```python
from build123d import *

# Parameters (mm, degrees)
SKETCH1_W           = 50
SKETCH1_H           = 53
BOSS_EXTRUDE1_DEPTH = 0.75
BOSS_EXTRUDE2_DEPTH = 1.5
SKETCH7_R           = 2
SKETCH7_R_2         = 1.948313055
CUT_EXTRUDE1_DEPTH  = 39.581083448
SKETCH8_W           = 21
SKETCH8_H           = 2.5
SKETCH8_W_2         = 6
SKETCH8_H_2         = 21
SKETCH8_W_3         = 16
BOSS_EXTRUDE3_DEPTH = 9
SKETCH9_R           = 2
BOSS_EXTRUDE4_DEPTH = 6
SKETCH10_W          = 14.5
SKETCH10_H          = 9
BOSS_EXTRUDE5_DEPTH = 11
SKETCH11_W          = 10
SKETCH11_H          = 7
BOSS_EXTRUDE6_DEPTH = 4
SKETCH12_W          = 6
SKETCH12_H          = 8
BOSS_EXTRUDE7_DEPTH = 6
SKETCH13_W          = 5
SKETCH13_H          = 12
BOSS_EXTRUDE8_DEPTH = 8
FILLET4_R           = 1
FILLET5_R           = 1


with BuildPart() as part:
    # Sketch1 → Boss-Extrude1 (new, symmetric)
    with BuildSketch(Plane(origin=(0, 0, 0), x_dir=(1, 0, 0), z_dir=(0, 1, 0))):
        Rectangle(SKETCH1_W, SKETCH1_H)
    extrude(amount=BOSS_EXTRUDE1_DEPTH, both=True)


with BuildPart() as body_2:
    # Sketch3 → Boss-Extrude2 (new body)
    with BuildSketch(Plane(origin=(0, 0.75, 0), x_dir=(1, 0, 0), z_dir=(0, 1, 0))):
        Polygon((25, -22.246887694), (25, 14.753112306), (28, 13.047029226), (28, -19.952970774), align=None)
    extrude(amount=-BOSS_EXTRUDE2_DEPTH)


with BuildPart() as cut_extrude1_tool:
    # Sketch7 → Cut-Extrude1 (new, through all)
    with BuildSketch(Plane(origin=(0, 0.75, 0), x_dir=(1, 0, 0), z_dir=(0, 1, 0))):
        with Locations(Location((-22.5, 24, 0), (0, 0, 270))):
            Circle(SKETCH7_R)
        with Locations(Location((-22.5, -24, 0), (0, 0, 270))):
            Circle(SKETCH7_R)
        with Locations((25, 11.753112306)):
            Circle(SKETCH7_R_2)
        with Locations((25, -19.246887694)):
            Circle(SKETCH7_R)
    extrude(amount=-CUT_EXTRUDE1_DEPTH)


with BuildPart() as part_1:
    add(part.part)

    # Cut-Extrude1: cut by cut_extrude1_tool
    add(cut_extrude1_tool.part, mode=Mode.SUBTRACT)



with BuildPart() as body_2_1:
    add(body_2.part)

    # Cut-Extrude1: cut by cut_extrude1_tool
    add(cut_extrude1_tool.part, mode=Mode.SUBTRACT)


with BuildPart() as part_2:
    add(part_1.part)

    add(body_2_1.part)  # Boss-Extrude3 merges body 2
    # Sketch8 → Boss-Extrude3 (add)
    with BuildSketch(Plane(origin=(0, 0.75, 0), x_dir=(1, 0, 0), z_dir=(0, 1, 0))):
        with Locations((13.5, 24.25)):
            Rectangle(SKETCH8_W, SKETCH8_H)
        with Locations((-8.5, 24.25)):
            Rectangle(SKETCH8_W, SKETCH8_H)
        with Locations((24, -5)):
            Rectangle(SKETCH8_W_2, SKETCH8_H_2)
        with Locations((15, -24.25)):
            Rectangle(SKETCH8_W_3, SKETCH8_H)
        with Locations((-3, -24.25)):
            Rectangle(SKETCH8_W_3, SKETCH8_H)
    extrude(amount=BOSS_EXTRUDE3_DEPTH)

    # Sketch9 → Boss-Extrude4 (add)
    with BuildSketch(Plane(origin=(0, 0.75, 0), x_dir=(1, 0, 0), z_dir=(0, 1, 0))):
        with Locations(Location((-2, -19, 0), (0, 0, 270))):
            Circle(SKETCH9_R)
        with Locations(Location((-2, -14.5, 0), (0, 0, 270))):
            Circle(SKETCH9_R)
        with Locations(Location((-8, -14.5, 0), (0, 0, 270))):
            Circle(SKETCH9_R)
    extrude(amount=BOSS_EXTRUDE4_DEPTH)

    # Sketch10 → Boss-Extrude5 (add)
    with BuildSketch(Plane(origin=(0, 0.75, 0), x_dir=(1, 0, 0), z_dir=(0, 1, 0))):
        with Locations((-20.75, -14)):
            Rectangle(SKETCH10_W, SKETCH10_H)
    extrude(amount=BOSS_EXTRUDE5_DEPTH)

    # Sketch11 → Boss-Extrude6 (add)
    with BuildSketch(Plane(origin=(0, 0.75, 0), x_dir=(1, 0, 0), z_dir=(0, 1, 0))):
        with Locations((-21, -1)):
            Rectangle(SKETCH11_W, SKETCH11_H)
    extrude(amount=BOSS_EXTRUDE6_DEPTH)

    # Sketch12 → Boss-Extrude7 (add)
    with BuildSketch(Plane(origin=(0, 0.75, 0), x_dir=(1, 0, 0), z_dir=(0, 1, 0))):
        with Locations((-21, 11.5)):
            Rectangle(SKETCH12_W, SKETCH12_H)
    extrude(amount=BOSS_EXTRUDE7_DEPTH)

    # Sketch13 → Boss-Extrude8 (add)
    with BuildSketch(Plane(origin=(0, 0.75, 0), x_dir=(1, 0, 0), z_dir=(0, 1, 0))):
        with Locations((-8.5, 8.5)):
            Rectangle(SKETCH13_W, SKETCH13_H)
    extrude(amount=BOSS_EXTRUDE8_DEPTH)

    # Fillet4
    fillet4_edges = [part_2.edges().sort_by_distance(p)[0] for p in [
        (-25, 0, -26.5),
    ]]
    fillet(fillet4_edges, radius=FILLET4_R)

    # Fillet5
    fillet5_edges = [part_2.edges().sort_by_distance(p)[0] for p in [
        (-25, 0, 26.5),
    ]]
    fillet(fillet5_edges, radius=FILLET5_R)


solid = part_2.part
```
Can you work these out from the model? Positions are in its coordinate system, mm. A direction names the side the tool comes from. Round coordinates to 2 decimals unless told otherwise and drop trailing zeros. Loops run counter-clockwise (first coordinate to the right, second up) from the corner with the lowest first, then second, coordinate; pieces in that order, holes last. Notation, with made-up numbers: (0, 63.5) -> (29, 63.5) arc R30 ccw to (29, 102.5) -> close; hole circle Ø6 at (-31, 18). An arc over 180 degrees is marked (long way). One line per item, written item: value. Start each with the question number.
1. If we section it at C-C, the plane z = 11.5: Write out the boundary of the cut face in (x, y), then the cut area to 3 significant figures.
2. For faces 1 (the flat face through (13, 5, -23)), 2 (the flat face through (-9, 9.75, -24)), 3 (the flat face through (3, 5, -24)), 4 (the flat face through (-21, 6, 18.5)), 5 (the flat face through (-9, 5, -14.5)), which set-ups out of +Z, -Z, +X, -X, +Y, -Y let a thin tool reach every point of the face, with its end or its side?
3. If we section it at B-B, the plane z = -24: Write out the boundary of the cut face in (x, y), then the cut area to 3 significant figures.
4. If we mould it in two halves opening along Z, with no side actions, what happens to faces 6 (the flat face through (-9, 5, -25.5)), 7 (the flat face through (13, 9.75, -24)), 8 (the flat face through (-6, 5, -8))? For each: pulls with the +Z half, pulls with the -Z half, needs draft (parallel to the pull), parting line crosses it, or undercut.
5. If I drill on probe 1 along Z at (x, y) = (22, 2.25); probe 2 along X at (y, z) = (4, -10); probe 3 along X at (y, z) = (3.25, 1.5), over which ranges is the centre line in solid material (lowest first)?
6. For pin 1 (1.8 mm diameter, centred on x = 24.5, z = 2, fed in from +Y); pin 2 (2 mm diameter, centred on x = -2.5, z = 19.5, fed in from +Y); pin 3 (4 mm diameter, centred on x = 16, y = 5, fed in from +Z), each with a flat end and sliding along its axis, tell me the tip position at first contact or that it passes through.
7. If we section it at D-D, the plane x = 15.5: Write out the boundary of the cut face in (y, z), then the cut area to 4 significant figures.
8. If we section it at A-A, the plane x = -22.5: Write out the boundary of the cut face in (y, z), then the cut area to 4 significant figures.
Calculated:
1. outline: (-28, 0.75) -> (-25, 0.75) -> (-25, -0.75) -> (28, -0.75) -> (28, 0.75) -> (27, 0.75) -> (27, 9.75) -> (21, 9.75) -> (21, 0.75) -> (-13.5, 0.75) -> (-13.5, 11.75) -> (-28, 11.75) -> close
1. area: 293 mm²
2. face 1: +X, -X, +Y
2. face 2: -Z, +X, -X, +Y
2. face 3: -Z, +Y
2. face 4: +Z, -X, +Y
2. face 5: +X, +Y
3. outline: (-25, -0.75) -> (-24.5, -0.75) -> (-24.5, 0.75) -> (-25, 0.75) -> close; (-20.5, -0.75) -> (25, -0.75) -> (25, 0.75) -> (24, 0.75) -> (24, 9.75) -> (3, 9.75) -> (3, 0.75) -> (2, 0.75) -> (2, 9.75) -> (-19, 9.75) -> (-19, 0.75) -> (-20.5, 0.75) -> close
3. area: 447 mm²
4. face 6: pulls with the -Z half
4. face 7: needs draft
4. face 8: undercut
5. probe 1: z = -25.5 to -23, -5.5 to 15.5, 23 to 25.5
5. probe 2: x = -24 to -18, -11 to -6
5. probe 3: x = -26 to -16, 21 to 27
6. pin 1: stops at y = 9.75
6. pin 2: stops at y = 6.75
6. pin 3: stops at z = 25.5
7. outline: (-0.75, -26.5) -> (0.75, -26.5) -> (0.75, -25.5) -> (9.75, -25.5) -> (9.75, -23) -> (0.75, -23) -> (0.75, 23) -> (9.75, 23) -> (9.75, 25.5) -> (0.75, 25.5) -> (0.75, 26.5) -> (-0.75, 26.5) -> close
7. area: 124.5 mm²
8. outline: (-0.75, -26.5) -> (0.75, -26.5) -> (0.75, -26) -> (-0.75, -26) -> close; (-0.75, -22) -> (0.75, -22) -> (0.75, -15.5) -> (6.75, -15.5) -> (6.75, -7.5) -> (0.75, -7.5) -> (0.75, -2.5) -> (4.75, -2.5) -> (4.75, 4.5) -> (0.75, 4.5) -> (0.75, 9.5) -> (11.75, 9.5) -> (11.75, 18.5) -> (0.75, 18.5) -> (0.75, 22) -> (-0.75, 22) -> close; (-0.75, 26) -> (0.75, 26) -> (0.75, 26.5) -> (-0.75, 26.5) -> close
8. area: 242.5 mm²
